from build123d import *

# Parameters (mm, degrees)
Y_KSEKLIK_EKSTR_ZYON1_DEPTH      = 13
IZIM1_2_R                        = 1.5
Y_KSEKLIK_EKSTR_ZYON2_DEPTH      = 2
IZIM1_4_R                        = 2.5
IZIM1_4_R_2                      = 1.5
Y_KSEKLIK_EKSTR_ZYON3_DEPTH      = 0.8
Y_KSEKLIK_EKSTR_ZYON4_DEPTH      = 3
DAIRESEL_KAPLAMA1_COUNT          = 4
Y_KSEKLIK_EKSTR_ZYON5_DEPTH      = 3
Y_KSEKLIK_EKSTR_ZYON5_DEPTH_BACK = 8.2
IZIM7_R                          = 1
IZIM1_6_R                        = 3
KES_EKSTR_ZYON2_DEPTH            = 15
IZIM1_7_R                        = 1.5
KES_EKSTR_ZYON3_DEPTH            = 3
KES_EKSTR_ZYON4_START            = 0.2
IZIM1_8_R                        = 4
IZIM1_8_R_2                      = 2.5
KES_EKSTR_ZYON4_DEPTH            = 0.2


with BuildPart() as part:
    # izim1 → Y_kseklik-Ekstr_zyon1 (new body)
    with BuildSketch(Plane.XY):
        with BuildLine():
            ThreePointArc((-10.274965018, 5.164793693), (9.2, -6.9), (-7.83519215, 8.417824183))
            ThreePointArc((-7.83519215, 8.417824183), (-8.419858501, 6.314893876), (-10.274965018, 5.164793693))
        make_face()
    y_kseklik_ekstr_zyon1 = extrude(amount=Y_KSEKLIK_EKSTR_ZYON1_DEPTH)

    # izim1_2 → Y_kseklik-Ekstr_zyon2 (add)
    with BuildSketch(Plane.XY):
        Circle(IZIM1_2_R)
    extrude(amount=-Y_KSEKLIK_EKSTR_ZYON2_DEPTH)

    # izim1_4 → Y_kseklik-Ekstr_zyon3 (add)
    with BuildSketch(Plane.XY):
        Circle(IZIM1_4_R)
        Circle(IZIM1_4_R_2, mode=Mode.SUBTRACT)
    extrude(amount=-Y_KSEKLIK_EKSTR_ZYON3_DEPTH)

    # izim5 → Y_kseklik-Ekstr_zyon4 (add, symmetric)
    with BuildSketch(Plane(origin=(0, 0, 0), x_dir=(0, 0, -1), z_dir=(1, 0, 0))):
        Polygon((-13, 11.5), (-18, 6.43916486), (-18, 0), (-15.732419213, 0), (-15.732419213, 6.806119772), (-13, 9.571784407), align=None)
    y_kseklik_ekstr_zyon4 = extrude(amount=Y_KSEKLIK_EKSTR_ZYON4_DEPTH, both=True)

    # Dairesel Kaplama1: Y_kseklik-Ekstr_zyon1, Y_kseklik-Ekstr_zyon4 ×4 about axis
    dairesel_kaplama1_axis = Axis((0, 0, 0), (0, 0, 1))
    add([y_kseklik_ekstr_zyon1.rotate(dairesel_kaplama1_axis, i * 360 / DAIRESEL_KAPLAMA1_COUNT) for i in range(1, DAIRESEL_KAPLAMA1_COUNT)])
    add([y_kseklik_ekstr_zyon4.rotate(dairesel_kaplama1_axis, i * 360 / DAIRESEL_KAPLAMA1_COUNT) for i in range(1, DAIRESEL_KAPLAMA1_COUNT)])

    # izim7 → Y_kseklik-Ekstr_zyon5 (add, two sides: drawn at the far end of the back side and taken through both)
    with BuildSketch(Plane.XY.offset(18).offset(-Y_KSEKLIK_EKSTR_ZYON5_DEPTH_BACK)):
        Circle(IZIM7_R)
    extrude(amount=Y_KSEKLIK_EKSTR_ZYON5_DEPTH + Y_KSEKLIK_EKSTR_ZYON5_DEPTH_BACK)

    # izim1_6 → Kes-Ekstr_zyon2 (cut)
    with BuildSketch(Plane.XY):
        with Locations((-10.819858501, 8.114893876)):
            Circle(IZIM1_6_R)
    extrude(amount=KES_EKSTR_ZYON2_DEPTH, mode=Mode.SUBTRACT)

    # izim1_7 → Kes-Ekstr_zyon3 (cut)
    with BuildSketch(Plane.XY):
        with Locations((-8, 0)):
            Circle(IZIM1_7_R)
        with Locations((0, 6)):
            Circle(IZIM1_7_R)
        with Locations((8, 0)):
            Circle(IZIM1_7_R)
        with Locations((0, -6)):
            Circle(IZIM1_7_R)
    extrude(amount=KES_EKSTR_ZYON3_DEPTH, mode=Mode.SUBTRACT)

    # izim1_8 → Kes-Ekstr_zyon4 (cut)
    with BuildSketch(Plane.XY.offset(KES_EKSTR_ZYON4_START)):
        Circle(IZIM1_8_R)
        Circle(IZIM1_8_R_2, mode=Mode.SUBTRACT)
    extrude(amount=-KES_EKSTR_ZYON4_DEPTH, mode=Mode.SUBTRACT)


solid = part.part
Can you work these out from the model? Positions are in its coordinate system, mm. A direction names the side the tool comes from. Coordinates: 2 decimals unless noted, no trailing zeros. Loops run counter-clockwise (first coordinate to the right, second up) from the corner with the lowest first, then second, coordinate; pieces in that order, holes last. Notation, with made-up numbers: (55, 51) - (113, 51) arc R19 cw to (113, 77) - close; hole circle Ø3 at (-34.75, 11). An arc over 180 degrees is marked (long way). Answer as a JSON object with one key per item and string values. Group by question number.
Item 1: If we section it at B-B (y = -6): List the corners of the cut face in (x, z) for me, plus the area to 3 significant figures.
Item 2: If I drill on L1, parallel to Y at x = 0, z = 0.15; L2, parallel to Z at x = 1, y = 4.75; L3, parallel to Z at x = -0.5, y = 6, over which ranges is the centre line in solid material (lowest first)? Write a range as from..to.
Item 3: If we section it at A-A (x = 8): List the corners of the cut face in (y, z) for me.
Item 4: If we section it at D-D (z = 14): List the corners of the cut face in (x, y) for me.
Item 5: For pin 1 (0.9 mm diameter, centred on x = -8.5, y = 0.5, fed in from -Z); pin 2 (1 mm diameter, centred on x = 7, y = -3, fed in from -Z); pin 3 (4 mm diameter, centred on x = -9, z = 18.5, fed in from +Y); pin 4 (4 mm diameter, centred on x = 8, z = 16.5, fed in from +Y), each with a flat end and sliding along its axis, tell me the tip position at first contact or that it passes through.
Item 6: On a 3-axis mill with a long thin cutter (end or side, diameter ignored), from which of +Z, -Z, +X, -X, +Y, -Y can I reach the whole of each face in a straight line? I mean faces 4 (the face through (0.042, 8.17, 14.385)), 5 (the face through (-3, 0, 13)), 6 (the face through (-3, 7, 16)), 7 (the face through (6.5, 0.07, 1.48)), 8 (the face through (-8.17, 0.042, 14.385)). Say none if no direction works.
Item 7: If we mould it in two halves opening along X, with no side actions, what happens to faces 1 (the face through (8.906, -7.276, 6.409)), 2 (the face through (5, 0, 0)), 3 (the face through (0.1, -1.4, 15.732))? For each: released by +X, released by -X, zero draft, split by the parting line, or undercut.
Item 8: If we section it at C-C (x = 2): List the corners of the cut face in (y, z) for me.
Returned:
{
 "1": {"outline": "(-9.81, 0) - (-1.5, 0) - (-1.5, 3) - (1.5, 3) - (1.5, 0) - (9.81, 0) - (9.81, 13) - (-9.81, 13) - close; (-3, 15.73) - (3, 15.73) - (3, 18) - (-3, 18) - close", "area": "260 mm²"},
 "2": {"L1": "y = -11.5..-7.5, -4.5..-4, -2.5..2.5, 4..4.5, 7.5..11.5", "L2": "z = 0..13, 15.73..18", "L3": "z = 3..13, 15.73..18"},
 "3": {"outline": "(-8.26, 0) - (-1.5, 0) - (-1.5, 3) - (1.5, 3) - (1.5, 0) - (8.26, 0) - (8.26, 13) - (-8.26, 13) - close; (-3, 14.55) - (3, 14.55) - (3, 16.46) - (-3, 16.46) - close"},
 "4": {"outline": "(-10.49, -3) - (-8.56, -3) - (-8.56, 3) - (-10.49, 3) - close; (-3, -10.49) - (3, -10.49) - (3, -8.56) - (-3, -8.56) - close; (-3, 8.56) - (3, 8.56) - (3, 10.49) - (-3, 10.49) - close; circle Ø2 at (0, 0); (8.56, -3) - (10.49, -3) - (10.49, 3) - (8.56, 3) - close"},
 "5": {"pin 1": "stops at z = 3", "pin 2": "stops at z = 0", "pin 3": "passes through", "pin 4": "stops at y = 3"},
 "6": {"face 4": "+X, -X", "face 5": "none", "face 6": "+Z, -X, +Y", "face 7": "-Z", "face 8": "+Y, -Y"},
 "7": {"face 1": "split by the parting line", "face 2": "zero draft", "face 3": "undercut"},
 "8": {"outline": "(-11.5, 13) - (-11.32, 13) - (-11.32, 0) - (-3.46, 0) - (-3.46, 0.2) - (-1.5, 0.2) - (-1.5, -0.8) - (1.5, -0.8) - (1.5, 0.2) - (3.46, 0.2) - (3.46, 0) - (11.32, 0) - (11.32, 13) - (11.5, 13) - (6.44, 18) - (-6.44, 18) - close; hole (-9.57, 13) - (9.57, 13) - (6.81, 15.73) - (-6.81, 15.73) - close"}
}
